Autodesk Inventor part; units mm, degrees
ref_plane "YZ Plane" through (0, 0, 0) normal (1, 0, 0) x (0, 1, 0)
ref_plane "XZ Plane" through (0, 0, 0) normal (0, 1, 0) x (-1, 0, 0)
ref_plane "XY Plane" through (0, 0, 0) normal (0, 0, 1) x (1, 0, 0)
sketch "Sketch1" plane through (0, 0, 0) normal (0, 1, 0) x (-1, 0, 0)
  line L0 (145, -100) -> (-145, -100)
  line L1 (-145, -100) -> (-145, 100)
  line L2 (-145, 100) -> (145, 100)
  line L3 (145, 100) -> (145, -100)
  line L4 (203, 0) -> (-203, 0)
  line L5 (0, -140) -> (0, 140)
  point P0 (0, 0)
  dimension "d30" = 290
  dimension "d31" = 200
extrude "Extrusion1" add sketch "Sketch1" along normal blind 6
sketch "Sketch2" plane through (0, 6, 0) normal (0, 1, 0) x (1, 0, 0)
  circle A0 centre (-19.75, -29.5) radius 13.5
  circle A1 centre (-82.75, -9.5) radius 13.5
  circle A2 centre (-19.75, 9.5) radius 13.5
  circle A3 centre (46.75, 29.5) radius 13.5
  circle A4 centre (82.75, 20.5) radius 13.5
  circle A5 centre (10.75, 29.5) radius 13.5
  circle A6 centre (10.75, -9.5) radius 13.5
  circle A7 centre (46.75, -9.5) radius 13.5
  circle A8 centre (82.75, -18.5) radius 13.5
  line L0 (-96.25, 43) -> (96.25, 43)
  line L1 (96.25, 43) -> (96.25, -43)
  line L2 (96.25, -43) -> (-96.25, -43)
  line L3 (-96.25, -43) -> (-96.25, 43)
  line L4 (145, 100) -> (-145, 100)
  line L5 (145, -100) -> (145, 100)
  line L6 (0, 140) -> (0, -140)
  line L7 (-203, 0) -> (203, 0)
  dimension "d3" = 27
  dimension "d19" = 30.5
  dimension "d20" = 36
  dimension "d23" = 19
  dimension "d24" = 9
  dimension "d25" = 36
  dimension "d26" = 11
  dimension "d27" = 9
  dimension "d28" = 11
  dimension "d29" = 63
extrude "Extrusion2" cut sketch "Sketch2" against normal blind 10 contours A0 | A8 | L6 A6 L7 | A6 L6 | A1 L7 | A1 L7 | A4 | A3 | A6 L7 | L7 A7 | A7 L7 | L6 A5 | A5 L6 | L7 A2 | A2 L7 picked at (6.7806, -6.3333)
fillet "Fillet1" radius 5 4 edges at (-145, 3, 100) (145, 3, 100) (145, 3, -100) (-145, 3, -100)
sketch "Sketch3" plane through (0, 6, 0) normal (0, 1, 0) x (1, 0, 0)
  circle A0 centre (-139.6667, 94.6667) radius 1.5
  line L0 (140, 100) -> (-140, 100)
  line L1 (-145, 95) -> (-145, -95)
  point P0 (0, 0)
  dimension "d35" = 5.3333
  dimension "d36" = 5.3333
  dimension "d37" = 3
extrude "Extrusion3" cut sketch "Sketch3" against normal blind 10
pattern_linear "Rectangular Pattern1" count 2 spacing 279.3333 along (1, 0, 0) count 2 spacing 189.3333 along (0, 0, 1) of "Extrusion3"
equation "\"d30\" = BoxLength"
equation "\"d31\" = BoxWidth"
equation "\"d0\" = SheetThickness"
equation "\"d3\" = button_hole_outer"
equation "\"d35\" = 0.666667 * CornerOffset + 0.333333 * SheetThickness"
equation "\"d36\" = 0.666667 * CornerOffset + 0.333333 * SheetThickness"
equation "\"d42\" = BoxLength - 1.33333 * CornerOffset - 0.666667 * SheetThickness"
equation "\"d45\" = BoxWidth - 1.33333 * CornerOffset - 0.666667 * SheetThickness"
equation "\"button_hole_outer\" = 27"
equation "\"BoxLength\" = 290"
equation "\"BoxWidth\" = 200"
equation "\"SheetThickness\" = 6"
equation "\"CornerOffset\" = 5"
properties part number "sega_straight"
CAD build for the part. Positions are in the model's coordinates, mm. Give positions to 0.01 mm unless a question says otherwise; leave off trailing zeros. Order: outer loops, then holes, each group sorted by start corner. A loop starts at its lowest first (then second) coordinate and runs counter-clockwise, first axis right, second up.
(1) Saw through at A-A, the plane x = -82.75. Give the cut face in (y, z).
(2) Saw through at B-B, the plane x = 82.75. Give the cut face in (y, z).
(3) Saw through at C-C, the plane z = -29.5. Give the cut face in (x, y).
(4) Drill centre lines: L1, parallel to Z at x = 46.75, y = 1.5; L2, parallel to Z at x = 84, y = 0.8; L3, parallel to X at y = 3.7, z = -9.5. Where is each one in solid material? Low to high.
(5) Saw through at D-D, the plane y = 3.4. State how many separate pieces and enclosed holes the cut face has, then the cut area to 3 significant figures.
(6) Mould opens along X. For faces 1 (the flat face through (145, 3, -1)), 2 (the cylindrical face through (43.82, 3.04, -16.32)), 3 (the flat face through (-2, 3, -100)) say: released by +X, released by -X, zero draft, split by the parting line, or undercut.
Results found:
1. outline: (0, -100) - (6, -100) - (6, -4) - (0, -4) - close; (0, 23) - (6, 23) - (6, 100) - (0, 100) - close
2. outline: (0, -100) - (6, -100) - (6, -34) - (0, -34) - close; (0, -7) - (6, -7) - (6, 5) - (0, 5) - close; (0, 32) - (6, 32) - (6, 100) - (0, 100) - close
3. outline: (-145, 0) - (-2.75, 0) - (-2.75, 6) - (-145, 6) - close; (24.25, 0) - (33.25, 0) - (33.25, 6) - (24.25, 6) - close; (60.25, 0) - (72.69, 0) - (72.69, 6) - (60.25, 6) - close; (92.81, 0) - (145, 0) - (145, 6) - (92.81, 6) - close
4. L1: z = -100 to -43, -16 to -4, 23 to 100
4. L2: z = -100 to -33.94, -7.06 to 5.06, 31.94 to 100
4. L3: x = -145 to -33.25, -6.25 to 74.92, 90.58 to 145
5. separate pieces: 1
5. enclosed holes: 13
5. area: 52,800 mm2
6. face 1: released by +X
6. face 2: undercut
6. face 3: zero draft
